For this review, take the finished solid that the model builds, in its own axes (mm). Face numbers are marked on the shaded views. A direction names the side the tool comes from. Coordinates: 2 decimals unless noted, no trailing zeros. Loops run counter-clockwise (first coordinate to the right, second up) from the corner with the lowest first, then second, coordinate; pieces in that order, holes last. Notation, with made-up numbers: (13, 45) -> (49, 45) arc R19 ccw to (49, 59) -> close; hole circle Ø4 at (72.5, 0). An arc over 180 degrees is marked (long way). One line per item, written item: value.
from build123d import *

# Parameters (mm, degrees)
SKETCH1_R               = 35
BOSS_EXTRUDE1_DEPTH     = 10
SKETCH2_R               = 23.5
BOSS_EXTRUDE2_DEPTH     = 13
BOSS_EXTRUDE3_DEPTH     = 4
SKETCH4_R               = 1.5
CUT_EXTRUDE1_DEPTH      = 4
MIRROR2_COPY_1_SKETCH_R = 1.5
MIRROR2_COPY_1_DEPTH    = 4
BOSS_EXTRUDE4_DEPTH     = 3
FILLET1_R               = 2
FILLET1_OF_MIRROR3_R    = 2
SKETCH6_W               = 14
SKETCH6_H               = 26
BOSS_EXTRUDE5_DEPTH     = 3
SKETCH7_R               = 10
CUT_EXTRUDE2_DEPTH      = 10


with BuildPart() as part:
    # Sketch1 → Boss-Extrude1 (new body)
    with BuildSketch(Plane(origin=(0, 0, 0), x_dir=(0, 0, -1), z_dir=(1, 0, 0))):
        Circle(SKETCH1_R)
    extrude(amount=BOSS_EXTRUDE1_DEPTH)

    # Sketch2 → Boss-Extrude2 (add)
    with BuildSketch(Plane(origin=(10, 0, 0), x_dir=(0, 0, -1), z_dir=(1, 0, 0))):
        with Locations(Location((0, 0, 0), (0, 0, 180))):
            Circle(SKETCH2_R)
    extrude(amount=BOSS_EXTRUDE2_DEPTH)

    # Sketch3 → Boss-Extrude3 (add)
    with BuildSketch(Plane(origin=(0, 13, 0), x_dir=(1, 0, 0), z_dir=(0, 1, 0))):
        Polygon((23, 35), (23, -35), (30.392057511, -43.809511096), (35.392057511, -43.809511096), (52.433760781, -23.5), (52.433760781, 23.5), (35.392057511, 43.809511096), (30.392057511, 43.809511096), align=None)
    boss_extrude3 = extrude(amount=-BOSS_EXTRUDE3_DEPTH)

    # Sketch4 → Cut-Extrude1 (cut)
    with BuildSketch(Plane(origin=(0, 13, 0), x_dir=(1, 0, 0), z_dir=(0, 1, 0))):
        with Locations(Location((32.892057511, -40.809511096, 0), (0, 0, 270))):
            Circle(SKETCH4_R)
    cut_extrude1 = extrude(amount=-CUT_EXTRUDE1_DEPTH, mode=Mode.SUBTRACT)

    # Mirror1: Cut-Extrude1 across plane
    add(cut_extrude1.mirror(Plane.XY), mode=Mode.SUBTRACT)

    # Mirror2: Boss-Extrude3, Cut-Extrude1 across plane
    add(boss_extrude3.mirror(Plane.ZX))
    add(cut_extrude1.mirror(Plane.ZX), mode=Mode.SUBTRACT)

    # Mirror2 copy 1 sketch → Mirror2 copy 1 (cut)
    with BuildSketch(Plane.XZ.offset(13)):
        with Locations(Location((32.892057511, -40.809511096, 0), (0, 0, 270))):
            Circle(MIRROR2_COPY_1_SKETCH_R)
    extrude(amount=-MIRROR2_COPY_1_DEPTH, mode=Mode.SUBTRACT)

    # Sketch5 → Boss-Extrude4 (add)
    with BuildSketch(Plane(origin=(23, 0, 0), x_dir=(0, 0, -1), z_dir=(1, 0, 0))):
        Polygon((0, 13), (-2, 13), (-2, 22), (2, 22), (2, 13), align=None)
    boss_extrude4 = extrude(amount=BOSS_EXTRUDE4_DEPTH)

    # Fillet1
    fillet1_edges = [part.edges().sort_by_distance(p)[0] for p in [
        (24.5, 22, 2),
        (24.5, 22, -2),
    ]]
    fillet(fillet1_edges, radius=FILLET1_R - 0.0001)  # a hair under: the kernel refuses the full size

    # Mirror3: Boss-Extrude4 across plane
    add(boss_extrude4.mirror(Plane.ZX))

    # Fillet1 of Mirror3
    fillet1_of_mirror3_edges = [part.edges().sort_by_distance(p)[0] for p in [
        (24.5, -22, 2),
        (24.5, -22, -2),
    ]]
    fillet(fillet1_of_mirror3_edges, radius=FILLET1_OF_MIRROR3_R - 0.0001)  # a hair under: the kernel refuses the full size

    # Sketch6 → Boss-Extrude5 (add)
    with BuildSketch(Plane(origin=(52.433760781, 0, 0), x_dir=(0, 0, -1), z_dir=(1, 0, 0))):
        Rectangle(SKETCH6_W, SKETCH6_H)
    extrude(amount=BOSS_EXTRUDE5_DEPTH)

    # Sketch7 → Cut-Extrude2 (cut)
    with BuildSketch(Plane.ZY):
        Circle(SKETCH7_R)
    extrude(amount=-CUT_EXTRUDE2_DEPTH, mode=Mode.SUBTRACT)


solid = part.part
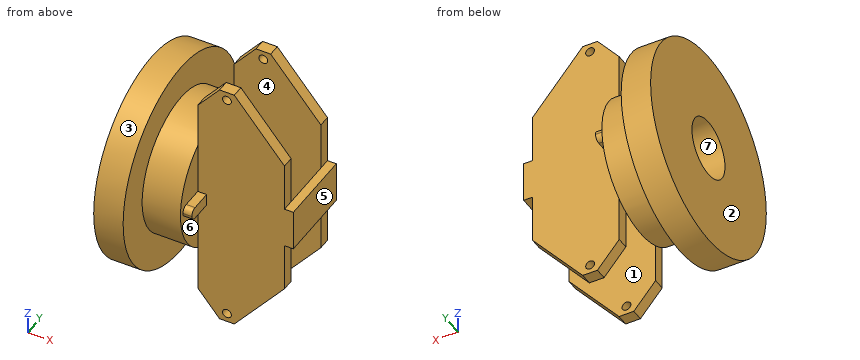
1. Take a section at A-A, the plane y = 0. Give the boundary of the cut face in (x, z), and give its area (3 significant figures).
Return value:
outline: (0, -35) -> (10, -35) -> (10, -23.5) -> (23, -23.5) -> (23, 23.5) -> (10, 23.5) -> (10, 35) -> (0, 35) -> (0, 10) -> (10, 10) -> (10, -10) -> (0, -10) -> close; (52.43, -7) -> (55.43, -7) -> (55.43, 7) -> (52.43, 7) -> close
area: 1,150 mm2
2. Insertion check: pin 1 Ø1.2 at (y, z) = (-11, 12) entering from +X; pin 2 Ø4 at (x, z) = (32.89, 40.81) entering from +Y; pin 3 Ø0.9 at (x, y) = (54, 0.5) entering from -Z. Each pin has a flat end and moves straight along its axis. Give the tip position at first contact, or say it passes through.
Return value:
pin 1: stops at x = 52.43
pin 2: stops at y = 13
pin 3: stops at z = -7
3. To check wall thickness, follow probe 1 along X at (y, z) = (3, -4); probe 2 along Y at (x, z) = (27, -15); probe 3 along X at (y, z) = (12, -23). State the ranges of each line that lie inside material, in increasing order. Write a range as from..to.
Return value:
probe 1: x = 10..23, 52.43..55.43
probe 2: y = -13..-9, 9..13
probe 3: x = 0..10, 23..52.43
4. The part is to be moulded in two halves that separate along X. For the marked faces 1, 2, 3 and 4, say which applies: pulls with the +X half, pulls with the -X half, needs draft (parallel to the pull), parting line crosses it, or undercut.
Return value:
face 1: undercut
face 2: pulls with the -X half
face 3: needs draft
face 4: undercut
5. Take a section at D-D, the plane z = -5. Give the boundary of the cut face in (x, y).
Return value:
outline: (0, -34.64) -> (10, -34.64) -> (10, -22.96) -> (23, -22.96) -> (23, -13) -> (55.43, -13) -> (55.43, 13) -> (23, 13) -> (23, 22.96) -> (10, 22.96) -> (10, 34.64) -> (0, 34.64) -> (0, 8.66) -> (10, 8.66) -> (10, -8.66) -> (0, -8.66) -> close; hole (23, -9) -> (52.43, -9) -> (52.43, 9) -> (23, 9) -> close
6. Take a section at B-B, the plane z = -29.5. Give the boundary of the cut face in (x, y).
Return value:
outline: (0, -18.83) -> (10, -18.83) -> (10, 18.83) -> (0, 18.83) -> close; (23, -13) -> (47.4, -13) -> (47.4, -9) -> (23, -9) -> close; (23, 9) -> (47.4, 9) -> (47.4, 13) -> (23, 13) -> close
7. For the marked faces 5, 6 and 7, list the 3-axis set-ups (+Z, -Z, +X, -X, +Y, -Y) from which the entire face can be reached by the end or side of a thin tool; tool diameter is ignored.
Return value:
face 5: +Z, -Z, +X, +Y, -Y
face 6: +X, -Y
face 7: -X
8. Take a section at C-C, the plane x = 43.5. Give the boundary of the cut face in (y, z), and give its area (3 significant figures).
Return value:
outline: (-13, -34.15) -> (-9, -34.15) -> (-9, 34.15) -> (-13, 34.15) -> close; (9, -34.15) -> (13, -34.15) -> (13, 34.15) -> (9, 34.15) -> close
area: 546 mm2
